Source: CAD feature listing. Evaluate the final solid. Frame: model axes, mm. A direction names the side the tool comes from. Give positions to 0.01 mm unless a question says otherwise; leave off trailing zeros. Order: outer loops, then holes, each group sorted by start corner. A loop starts at its lowest first (then second) coordinate and runs counter-clockwise, first axis right, second up. Notation, with made-up numbers: (-14.5, -15) - (-9.5, -15) arc R28 cw to (-9.5, 20) - close; hole circle Ø2 at (70.25, 70.25). An arc over 180 degrees is marked (long way). Use CSV: the item, a comma, the result in double quotes.
Autodesk Fusion 360 part; units mm, degrees
sketch "Sketch1" plane through (0, 0, 0) normal (0, 0, 1) x (1, 0, 0) in component "Spacer"
  line L0 (0, 0) -> (35, 0)
  line L1 (35, 0) -> (35, 15)
  line L2 (35, 15) -> (0, 15)
  line L3 (0, 15) -> (0, 0)
  line L4 (0, 65) -> (35, 65)
  line L5 (35, 65) -> (35, 80)
  line L6 (35, 80) -> (0, 80)
  line L7 (0, 80) -> (0, 65)
  line L8 (35, 0) -> (40, 0)
  line L9 (40, 0) -> (40, 80)
  line L10 (40, 80) -> (35, 80)
  line L11 (35, 80) -> (35, 0)
  dimension "d1" = 35
  dimension "d2" = 15
  dimension "d3" = 35
  dimension "d4" = 15
  dimension "d5" = 50
  dimension "d6" = 35
  dimension "d7" = 5
  dimension "d8" = 80
extrude "Extrude1" add sketch "Sketch1" along normal blind 70 contours L0 L1 L2 L3 L11 | L4 L5 L6 L7 L11 makes body 1 at (23.3333, 15, 46.6667) makes body 2 at (11.6667, 65, 46.6667) in component "Spacer"
extrude "Extrude2" add sketch "Sketch1" along normal blind 20 contours L1 L5 L8 L9 L10 L11 bodies 1 2 in component "Spacer"
fillet "Fillet1" radius 2 3 edges at (40, 40, 20) (40, 0, 10) (40, 80, 10) on bodies 1 in component "Spacer"
fillet "Fillet2" radius 3 2 edges at (0, 72.5, 70) (0, 7.5, 70) on bodies 1 in component "Spacer"
component "Spacer" placed x (1, 0, 0) y (0, 1, 0) z (0, 0, 1) at (0, 0, 0)
Item 1: Set-up query: faces 4 (the flat face through (35, 40, 10)), 5 (the flat face through (19, 0, 35)), 6 (the flat face through (35, 7, 45)). Return all of +Z, -Z, +X, -X, +Y, -Y with unobstructed straight access to the full face (end or side cutting, diameter ignored); none if empty.
Filled in:
face 4,"+Z, -Z, -X"
face 5,"+Z, -Z, +X, -X, -Y"
face 6,"+Z, +X, +Y, -Y"
Item 2: Section C-C on y = 71.5. Return the cut outline in (x, z), then the cut area to 3 significant figures.
Filled in:
outline,"(0, 0) - (40, 0) - (40, 18) arc R2 ccw to (38, 20) - (35, 20) - (35, 70) - (3, 70) arc R3 ccw to (0, 67) - close"
area,"2,550 mm2"
Item 3: Section D-D on z = 15. Return the cut outline in (x, y).
Filled in:
outline,"(0, 0) - (38, 0) arc R2 ccw to (40, 2) - (40, 78) arc R2 ccw to (38, 80) - (0, 80) - (0, 65) - (35, 65) - (35, 15) - (0, 15) - close"
Item 4: Material intervals for line 1 (Y direction, x = 5, z = 61); line 2 (X direction, y = 13, z = 25.5); line 3 (X direction, y = 18, z = 13.5), sorted ascending. Write a range as from..to.
Filled in:
line 1,"y = 0..15, 65..80"
line 2,"x = 0..35"
line 3,"x = 35..40"
Item 5: Section A-A on x = 21.5. Return the cut outline in (y, z).
Filled in:
outline,"(0, 0) - (15, 0) - (15, 70) - (0, 70) - close; (65, 0) - (80, 0) - (80, 70) - (65, 70) - close"
Item 6: Section B-B on z = 30. Return the cut outline in (x, y).
Filled in:
outline,"(0, 0) - (35, 0) - (35, 15) - (0, 15) - close; (0, 65) - (35, 65) - (35, 80) - (0, 80) - close"
Item 7: First-contact query: pin 1 (16 mm diameter, centred on y = 28.5, z = 10, fed in from -X); pin 2 (1.5 mm diameter, centred on x = 37, y = 33.5, fed in from +Z); pin 3 (12 mm diameter, centred on y = 5, z = 35, fed in from +X). Flat tips, straight axial feed; report the tip coordinate or a pass-through.
Filled in:
pin 1,"stops at x = 35"
pin 2,"stops at z = 20"
pin 3,"stops at x = 35"
Item 8: Mould query, pull axis Y, two halves, no side actions, for faces 1 (the flat face through (19, 8, 70)), 2 (the flat face through (18, 15, 35)), 3 (the cylindrical face through (39.4, 0.57, 10.14)). Classes: released by +Y, released by -Y, zero draft, split by the parting line, or undercut.
Filled in:
face 1,"zero draft"
face 2,"undercut"
face 3,"released by -Y"
